from build123d import *

# Parameters (mm, degrees)
ESBO_O1_W                 = 90
ESBO_O1_H                 = 10
RESSALTO_EXTRUS_O1_DEPTH  = 100
CORTE_EXTRUS_O1_DEPTH     = 73
ESBO_O5_W                 = 11
ESBO_O5_H                 = 6.5
CORTE_EXTRUS_O2_DEPTH     = 135.907375632
ESBO_O8_W                 = 94
ESBO_O8_H                 = 5
CORTE_EXTRUS_O3_DEPTH     = 3
ESBO_O9_W                 = 94
ESBO_O9_H                 = 84
RESSALTO_EXTRUS_O2_DEPTH  = 8
ESBO_O10_W                = 34
ESBO_O10_H                = 18
CORTE_EXTRUS_O4_DEPTH     = 22
ESBO_O11_W                = 34
ESBO_O11_H                = 18
CORTE_EXTRUS_O5_DEPTH     = 22
CORTE_EXTRUS_O8_DEPTH     = 100
ESBO_O19_W                = 53
ESBO_O19_H                = 0.919551387
CORTE_EXTRUS_O10_DEPTH    = 136.735036008
RESSALTO_EXTRUS_O4_DEPTH  = 56
ESBO_O21_W                = 3
ESBO_O21_H                = 3
RESSALTO_EXTRUS_O5_DEPTH  = 56
RESSALTO_EXTRUS_O6_DEPTH  = 100
ESBO_O25_R                = 1.5
CORTE_EXTRUS_O11_DEPTH    = 135.985184372
ESBO_O26_R                = 1.5
CORTE_EXTRUS_O14_DEPTH    = 135.985184372
ESBO_O28_W                = 3
ESBO_O28_H                = 51.10099753
RESSALTO_EXTRUS_O7_DEPTH  = 7
RESSALTO_EXTRUS_O8_DEPTH  = 62
ESBO_O30_W                = 16
ESBO_O30_H                = 3
RESSALTO_EXTRUS_O9_DEPTH  = 7
ESBO_O31_W                = 62
ESBO_O31_H                = 12
CORTE_EXTRUS_O15_DEPTH    = 7
ESBO_O33_W                = 3
ESBO_O33_H                = 3.919551387
RESSALTO_EXTRUS_O11_DEPTH = 22
ESBO_O34_W                = 3
ESBO_O34_H                = 3.919551387
RESSALTO_EXTRUS_O12_DEPTH = 22
ESBO_O35_W                = 19
ESBO_O35_H                = 0.080448613
RESSALTO_EXTRUS_O13_DEPTH = 3
ESBO_O36_R                = 1.5
CORTE_EXTRUS_O16_DEPTH    = 135.985184372
ESBO_O37_W                = 14
ESBO_O37_H                = 4
CORTE_EXTRUS_O17_DEPTH    = 6
RESSALTO_EXTRUS_O14_DEPTH = 100
ESBO_O39_R                = 1.5
ESBO_O39_R_2              = 1.500009338
CORTE_EXTRUS_O18_DEPTH    = 4
ESBO_O40_R                = 1.5
CORTE_EXTRUS_O19_DEPTH    = 10
CORTE_EXTRUS_O21_DEPTH    = 7
ESBO_O43_W                = 55
ESBO_O43_H                = 14.196322654
CORTE_EXTRUS_O23_DEPTH    = 2


with BuildPart() as part:
    # Esboço1 → Ressalto-extrusão1 (new body)
    with BuildSketch(Plane(origin=(0, 0, 0), x_dir=(0, 0, -1), z_dir=(1, 0, 0))):
        with Locations((45, 5)):
            Rectangle(ESBO_O1_W, ESBO_O1_H)
    extrude(amount=RESSALTO_EXTRUS_O1_DEPTH)

    # Esboço3 → Corte-extrusão1 (cut)
    with BuildSketch(Plane(origin=(0, 0, -90), x_dir=(-1, 0, 0), z_dir=(0, 0, -1))):
        Polygon((-93, 0), (-93, 2), (-97, 2), (-97, 7), (-3, 7), (-3, 2), (-7, 2), (-7, 0), align=None)
    extrude(amount=-CORTE_EXTRUS_O1_DEPTH, mode=Mode.SUBTRACT)

    # Esboço5 → Corte-extrusão2 (cut, through all)
    with BuildSketch(Plane(origin=(0, 10, 0), x_dir=(1, 0, 0), z_dir=(0, 1, 0))):
        with Locations((10.5, 9.25)):
            Rectangle(ESBO_O5_W, ESBO_O5_H)
        with Locations((89.5, 9.25)):
            Rectangle(ESBO_O5_W, ESBO_O5_H)
    extrude(amount=-CORTE_EXTRUS_O2_DEPTH, mode=Mode.SUBTRACT)

    # Esboço8 → Corte-extrusão3 (cut)
    with BuildSketch(Plane(origin=(0, 0, -17), x_dir=(-1, 0, 0), z_dir=(0, 0, -1))):
        with Locations((-50, 4.5)):
            Rectangle(ESBO_O8_W, ESBO_O8_H)
    extrude(amount=-CORTE_EXTRUS_O3_DEPTH, mode=Mode.SUBTRACT)

    # Esboço9 → Ressalto-extrusão2 (add)
    with BuildSketch(Plane(origin=(0, 10, 0), x_dir=(1, 0, 0), z_dir=(0, 1, 0))):
        Polygon((0, 1.678302474), (0, 0), (2, 0), (100, 0), (100, 1.678302474), (100, 90), (97, 90), (3, 90), (0, 90), align=None)
        with Locations((50, 45)):
            Rectangle(ESBO_O9_W, ESBO_O9_H, mode=Mode.SUBTRACT)
    extrude(amount=RESSALTO_EXTRUS_O2_DEPTH)

    # Esboço10 → Corte-extrusão4 (cut)
    with BuildSketch(Plane.ZY):
        with Locations((-73, 9)):
            Rectangle(ESBO_O10_W, ESBO_O10_H)
    extrude(amount=-CORTE_EXTRUS_O4_DEPTH, mode=Mode.SUBTRACT)

    # Esboço11 → Corte-extrusão5 (cut)
    with BuildSketch(Plane(origin=(100, 0, 0), x_dir=(0, 0, -1), z_dir=(1, 0, 0))):
        with Locations((73, 9)):
            Rectangle(ESBO_O11_W, ESBO_O11_H)
    extrude(amount=-CORTE_EXTRUS_O5_DEPTH, mode=Mode.SUBTRACT)

    # Esboço15 → Corte-extrusão8 (cut)
    with BuildSketch(Plane(origin=(100, 0, 0), x_dir=(0, 0, -1), z_dir=(1, 0, 0))):
        Polygon((0, 5.88429619), (3.246393052, 18), (0, 18), align=None)
    extrude(amount=-CORTE_EXTRUS_O8_DEPTH, mode=Mode.SUBTRACT)

    # Esboço19 → Corte-extrusão10 (cut, through all)
    with BuildSketch(Plane(origin=(100, 0, 0), x_dir=(0, 0, -1), z_dir=(1, 0, 0))):
        with Locations((29.5, 17.540224307)):
            Rectangle(ESBO_O19_W, ESBO_O19_H)
    extrude(amount=-CORTE_EXTRUS_O10_DEPTH, mode=Mode.SUBTRACT)

    # Esboço20 → Ressalto-extrusão4 (add)
    with BuildSketch(Plane(origin=(78, 0, 0), x_dir=(0, 0, -1), z_dir=(1, 0, 0))):
        with BuildLine():
            Line((68.839605241, 11), (77.137237802, 11))
            ThreePointArc((77.137237802, 11), (78.871318989, 13.239422392), (79.48840166, 16.003705155))
            Line((79.48840166, 16.003705155), (82.48840166, 16.003705155))
            Line((82.48840166, 16.003705155), (82.48840166, 14))
            Line((82.48840166, 14), (82.48840166, 13))
            Line((82.48840166, 13), (82.48840166, 10))
            Line((82.48840166, 10), (81.830476132, 10))
            Line((81.830476132, 10), (63.488441382, 10))
            Line((63.488441382, 10), (63.488441382, 14))
            Line((63.488441382, 14), (63.488441382, 16.003705155))
            Line((63.488441382, 16.003705155), (66.488441382, 16.003705155))
            ThreePointArc((66.488441382, 16.003705155), (67.105524053, 13.239422392), (68.839605241, 11))
        make_face()
    extrude(amount=-RESSALTO_EXTRUS_O4_DEPTH)

    # Esboço21 → Ressalto-extrusão5 (add)
    with BuildSketch(Plane(origin=(78, 0, 0), x_dir=(0, 0, -1), z_dir=(1, 0, 0))):
        with Locations((88.5, 19.5)):
            Rectangle(ESBO_O21_W, ESBO_O21_H)
    extrude(amount=-RESSALTO_EXTRUS_O5_DEPTH)

    # Esboço22 → Ressalto-extrusão6 (add)
    with BuildSketch(Plane(origin=(100, 0, 0), x_dir=(0, 0, -1), z_dir=(1, 0, 0))):
        Polygon((4.89900247, 17.080448613), (3, 10), (3, 17.080448613), align=None)
    extrude(amount=-RESSALTO_EXTRUS_O6_DEPTH)

    # Esboço25 → Corte-extrusão11 (cut, through all)
    with BuildSketch(Plane(origin=(0, 10, 0), x_dir=(1, 0, 0), z_dir=(0, 1, 0))):
        with Locations(Location((10.5, 28.335399636, 0), (0, 0, 270))):
            Circle(ESBO_O25_R)
    extrude(amount=-CORTE_EXTRUS_O11_DEPTH, mode=Mode.SUBTRACT)

    # Esboço26 → Corte-extrusão14 (cut, through all)
    with BuildSketch(Plane(origin=(0, 10, 0), x_dir=(1, 0, 0), z_dir=(0, 1, 0))):
        with Locations(Location((89.5, 28.335399636, 0), (0, 0, 270))):
            Circle(ESBO_O26_R)
    extrude(amount=-CORTE_EXTRUS_O14_DEPTH, mode=Mode.SUBTRACT)

    # Esboço28 → Ressalto-extrusão7 (add)
    with BuildSketch(Plane(origin=(0, 10, 0), x_dir=(1, 0, 0), z_dir=(0, 1, 0))):
        with Locations((20.5, 30.449501235)):
            Rectangle(ESBO_O28_W, ESBO_O28_H)
        with Locations((79.5, 30.449501235)):
            Rectangle(ESBO_O28_W, ESBO_O28_H)
    extrude(amount=RESSALTO_EXTRUS_O7_DEPTH)

    # Esboço29 → Ressalto-extrusão8 (add)
    with BuildSketch(Plane(origin=(81, 0, 0), x_dir=(0, 0, -1), z_dir=(1, 0, 0))):
        Polygon((4.89900247, 10), (3, 10), (4.89900247, 17.080448613), align=None)
    extrude(amount=-RESSALTO_EXTRUS_O8_DEPTH)

    # Esboço30 → Ressalto-extrusão9 (add)
    with BuildSketch(Plane(origin=(0, 17, 0), x_dir=(1, 0, 0), z_dir=(0, 1, 0))):
        with Locations((11, 54.5)):
            Rectangle(ESBO_O30_W, ESBO_O30_H)
        with Locations((89, 54.5)):
            Rectangle(ESBO_O30_W, ESBO_O30_H)
    extrude(amount=-RESSALTO_EXTRUS_O9_DEPTH)

    # Esboço31 → Corte-extrusão15 (cut)
    with BuildSketch(Plane(origin=(0, 17, 0), x_dir=(1, 0, 0), z_dir=(0, 1, 0))):
        with Locations((50, 47)):
            Rectangle(ESBO_O31_W, ESBO_O31_H)
    extrude(amount=-CORTE_EXTRUS_O15_DEPTH, mode=Mode.SUBTRACT)

    # Esboço33 → Ressalto-extrusão11 (add)
    with BuildSketch(Plane(origin=(100, 0, 0), x_dir=(0, 0, -1), z_dir=(1, 0, 0))):
        with Locations((54.5, 19.040224307)):
            Rectangle(ESBO_O33_W, ESBO_O33_H)
    extrude(amount=-RESSALTO_EXTRUS_O11_DEPTH)

    # Esboço34 → Ressalto-extrusão12 (add)
    with BuildSketch(Plane.ZY):
        with Locations((-54.5, 19.040224307)):
            Rectangle(ESBO_O34_W, ESBO_O34_H)
    extrude(amount=-RESSALTO_EXTRUS_O12_DEPTH)

    # Esboço35 → Ressalto-extrusão13 (add)
    with BuildSketch(Plane(origin=(0, 0, -56), x_dir=(-1, 0, 0), z_dir=(0, 0, -1))):
        with Locations((-12.5, 17.040224307)):
            Rectangle(ESBO_O35_W, ESBO_O35_H)
        with Locations((-87.5, 17.040224307)):
            Rectangle(ESBO_O35_W, ESBO_O35_H)
    extrude(amount=-RESSALTO_EXTRUS_O13_DEPTH)

    # Esboço36 → Corte-extrusão16 (cut, through all)
    with BuildSketch(Plane(origin=(0, 10, 0), x_dir=(1, 0, 0), z_dir=(0, 1, 0))):
        with Locations(Location((71.5, 61.233441382, 0), (0, 0, 270))):
            Circle(ESBO_O36_R)
        with Locations(Location((28.5, 61.233441382, 0), (0, 0, 270))):
            Circle(ESBO_O36_R)
        with Locations(Location((71.5, 84.74340166, 0), (0, 0, 270))):
            Circle(ESBO_O36_R)
        with Locations(Location((28.5, 84.74340166, 0), (0, 0, 270))):
            Circle(ESBO_O36_R)
    extrude(amount=-CORTE_EXTRUS_O16_DEPTH, mode=Mode.SUBTRACT)

    # Esboço37 → Corte-extrusão17 (cut)
    with BuildSketch(Plane.XY.offset(-63.488441382)):
        with Locations((50, 14.003705155)):
            Rectangle(ESBO_O37_W, ESBO_O37_H)
    extrude(amount=-CORTE_EXTRUS_O17_DEPTH, mode=Mode.SUBTRACT)

    # Esboço38 → Ressalto-extrusão14 (add, through all)
    with BuildSketch(Plane(origin=(100, 0, 0), x_dir=(0, 0, -1), z_dir=(1, 0, 0))):
        Polygon((0, 0), (-5.88429619, 0), (0, 5.88429619), align=None)
    extrude(amount=-RESSALTO_EXTRUS_O14_DEPTH)

    # Esboço39 → Corte-extrusão18 (cut)
    with BuildSketch(Plane(origin=(0, 0.394173103, 1.471074047), x_dir=(1, 0, 0), z_dir=(0, 0.258819045102519, 0.9659258262890689))):
        with Locations(Location((30, 12.950688916, 0), (0, 0, 270))):
            Circle(ESBO_O39_R)
        with Locations(Location((70, 12.950688916, 0), (0, 0, 270))):
            Circle(ESBO_O39_R_2)
    extrude(amount=-CORTE_EXTRUS_O18_DEPTH, mode=Mode.SUBTRACT)

    # Esboço40 → Corte-extrusão19 (cut)
    with BuildSketch(Plane.XZ):
        with Locations(Location((28.5, -10.233441382, 0), (0, 0, 270))):
            Circle(ESBO_O40_R)
        with Locations(Location((71.5, -10.233441382, 0), (0, 0, 270))):
            Circle(ESBO_O40_R)
    extrude(amount=-CORTE_EXTRUS_O19_DEPTH, mode=Mode.SUBTRACT)

    # Esboço42 → Corte-extrusão21 (cut)
    with BuildSketch(Plane(origin=(0, 0, -14), x_dir=(-1, 0, 0), z_dir=(0, 0, -1))):
        Polygon((-77.5, 7), (-22.5, 7), (-22.5, 2), (-22.5, 0), (-77.5, 0), (-77.5, 2), align=None)
    extrude(amount=-CORTE_EXTRUS_O21_DEPTH, mode=Mode.SUBTRACT)

    # Esboço43 → Corte-extrusão23 (cut)
    with BuildSketch(Plane.XZ):
        with Locations((50, -14.098161327)):
            Rectangle(ESBO_O43_W, ESBO_O43_H)
    extrude(amount=-CORTE_EXTRUS_O23_DEPTH, mode=Mode.SUBTRACT)


solid = part.part
Geometry: final body of the model. Coordinates: model frame, mm. A direction names the side the tool comes from. Give positions to 0.01 mm unless a question says otherwise; leave off trailing zeros. Write each loop counter-clockwise with the first axis right and the second up, starting at its lowest first coordinate (ties: lowest second). Pieces come first, ordered by that corner, then holes. Notation, with made-up numbers: M 38,13 L 92,13 A30 cw 92,36 Z; hole C -20,63 d8. An arc over 180 degrees is marked long. Answer in a Markdown table with one row per item. Add a question column.
(1) Section D-D on z = -74.5. Return loops of the section in (x, y), and give its area (3 significant figures).
(2) Mould query, pull axis Z, two halves, no side actions, for faces 5 (the flat face through (22.5, 3, -11)), 6 (the flat face through (89, 5, -6)), 7 (the flat face through (50, 14, -90)), 8 (the flat face through (5, 5, -9)). Classes: +Z half, -Z half, draft (parallel to the pull), parting line (faces both ways), or undercut.
(3) Section A-A on x = 89.5. Return loops of the section in (y, z).
(4) Reachability of faces 1 (the flat face through (77.5, 4, -11)), 2 (the flat face through (57, 14, -65)), 3 (the flat face through (16, 5, -9)), 4 (the flat face through (50.4, 11.6, -63.488)) from +Z, -Z, +X, -X, +Y, -Y: full face, straight path, thin tool, end or side. Return the list, or none.
(5) First-contact query: pin 1 (1.6 mm diameter, centred on x = 11, y = 0.5, fed in from -Z); pin 2 (3 mm diameter, centred on y = 14.5, z = -30.5, fed in from -X); pin 3 (6.5 mm diameter, centred on x = 7, y = 9.5, fed in from -Z); pin 4 (3 mm diameter, centred on x = 23, z = -21, fed in from -Y). Flat tips, straight axial feed; report the tip coordinate or a pass-through.
(6) Section C-C on x = 38. Return loops of the section in (y, z).
(7) Ray query, line 1 (X direction, y = 12.5, z = -14.5); line 2 (X direction, y = 5.5, z = -14.5); line 3 (X direction, y = 13.25, z = -3). Return the intervals inside material, ascending.
(8) Section B-B on z = -25.5. Return loops of the section in (x, y).
Result set:
| question | item | result |
|---|---|---|
| 1 | outline | M 22,7 L 78,7 L 78,11 L 22,11 Z |
| 1 | area | 224 mm^2 |
| 2 | face 5 | draft |
| 2 | face 6 | undercut |
| 2 | face 7 | -Z half |
| 2 | face 8 | undercut |
| 3 | outline | M 0,-17 L 2,-17 L 2,-14 L 7,-14 L 7,-26.84 L 10,-26.84 L 10,-12.5 L 0,-12.5 Z; M 0,-6 L 10,-6 L 10,-3 L 17.08,-4.9 L 17.08,-3 L 5.88,0 L 0,5.88 Z; M 7,-56 L 21,-56 L 21,-53 L 10,-53 L 10,-29.84 L 7,-29.84 Z |
| 4 | face 1 | -Z, -Y |
| 4 | face 2 | +Y |
| 4 | face 3 | +Y, -Y |
| 4 | face 4 | +X, -X, +Y |
| 5 | pin 1 | stops at z = -17 |
| 5 | pin 2 | stops at x = 0 |
| 5 | pin 3 | stops at z = -56 |
| 5 | pin 4 | stops at y = 7 |
| 6 | outline | M 0,-7 L 7,-7 L 7,-90 L 21,-90 L 21,-87 L 10,-87 L 10,-82.49 L 16,-82.49 L 16,-79.49 A6.5 cw 11,-77.14 L 11,-68.84 A6.5 cw 16,-66.49 L 16,-63.49 L 10,-63.49 L 10,-4.9 L 17.08,-4.9 L 17.08,-3 L 5.88,0 L 0,5.88 Z |
| 7 | line 1 | x = 0 to 3, 19 to 22, 78 to 81, 97 to 100 |
| 7 | line 2 | x = 0 to 3, 97 to 100 |
| 7 | line 3 | x = 0 to 28.64, 31.36 to 68.64, 71.36 to 100 |
| 8 | outline | M 0,0 L 7,0 L 7,2 L 3,2 L 3,7 L 97,7 L 97,2 L 93,2 L 93,0 L 100,0 L 100,17.08 L 97,17.08 L 97,10 L 81,10 L 81,17 L 78,17 L 78,10 L 22,10 L 22,17 L 19,17 L 19,10 L 3,10 L 3,17.08 L 0,17.08 Z |
